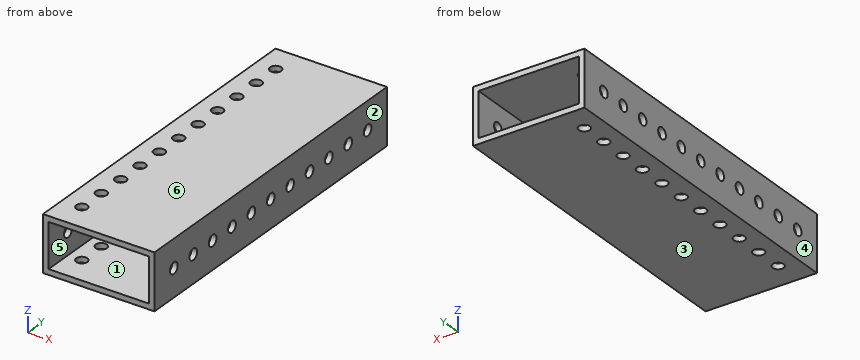
```python
from build123d import *

# Parameters (mm, degrees)
SKETCH1_W           = 50.8
SKETCH1_H           = 25.4
SKETCH1_W_2         = 45.72
SKETCH1_H_2         = 20.32
BOSS_EXTRUDE2_DEPTH = 152.4
SKETCH2_R           = 2.54
CUT_EXTRUDE1_DEPTH  = 127
SKETCH3_R           = 2.54
CUT_EXTRUDE2_DEPTH  = 166.725706651


with BuildPart() as part:
    # Sketch1 → Boss-Extrude2 (new body)
    with BuildSketch(Plane(origin=(0, 0, 0), x_dir=(1, 0, 0), z_dir=(0, 1, 0))):
        with Locations((-34.550728477, 5.021125828)):
            Rectangle(SKETCH1_W, SKETCH1_H)
        with Locations((-34.550728477, 5.021125828)):
            Rectangle(SKETCH1_W_2, SKETCH1_H_2, mode=Mode.SUBTRACT)
    extrude(amount=BOSS_EXTRUDE2_DEPTH)

    # Sketch2 → Cut-Extrude1 (cut)
    with BuildSketch(Plane(origin=(-9.150728477, 0, 0), x_dir=(0, 0, -1), z_dir=(1, 0, 0))):
        with Locations((5.021125828, 139.7)):
            Circle(SKETCH2_R)
        with Locations((5.021125828, 127)):
            Circle(SKETCH2_R)
        with Locations((5.021125828, 114.3)):
            Circle(SKETCH2_R)
        with Locations((5.021125828, 101.6)):
            Circle(SKETCH2_R)
        with Locations((5.021125828, 88.9)):
            Circle(SKETCH2_R)
        with Locations((5.021125828, 76.2)):
            Circle(SKETCH2_R)
        with Locations((5.021125828, 63.5)):
            Circle(SKETCH2_R)
        with Locations((5.021125828, 50.8)):
            Circle(SKETCH2_R)
        with Locations((5.021125828, 38.1)):
            Circle(SKETCH2_R)
        with Locations((5.021125828, 25.4)):
            Circle(SKETCH2_R)
        with Locations((5.021125828, 12.7)):
            Circle(SKETCH2_R)
    extrude(amount=-CUT_EXTRUDE1_DEPTH, mode=Mode.SUBTRACT)

    # Sketch3 → Cut-Extrude2 (cut, through all)
    with BuildSketch(Plane(origin=(0, 0, -17.721125828), x_dir=(-1, 0, 0), z_dir=(0, 0, -1))):
        with Locations((51.060728477, 139.7)):
            Circle(SKETCH3_R)
        with Locations((51.060728477, 127)):
            Circle(SKETCH3_R)
        with Locations((51.060728477, 114.3)):
            Circle(SKETCH3_R)
        with Locations((51.060728477, 101.6)):
            Circle(SKETCH3_R)
        with Locations((51.060728477, 88.9)):
            Circle(SKETCH3_R)
        with Locations((51.060728477, 76.2)):
            Circle(SKETCH3_R)
        with Locations((51.060728477, 63.5)):
            Circle(SKETCH3_R)
        with Locations((51.060728477, 50.8)):
            Circle(SKETCH3_R)
        with Locations((51.060728477, 38.1)):
            Circle(SKETCH3_R)
        with Locations((51.060728477, 25.4)):
            Circle(SKETCH3_R)
        with Locations((51.060728477, 12.7)):
            Circle(SKETCH3_R)
    extrude(amount=-CUT_EXTRUDE2_DEPTH, mode=Mode.SUBTRACT)


solid = part.part
```
The model under review builds one solid part; all positions refer to its coordinate system, in mm. Face numbers are marked on the shaded views. A direction names the side the tool comes from. Round coordinates to 2 decimals unless told otherwise and drop trailing zeros. Loops run counter-clockwise (first coordinate to the right, second up) from the corner with the lowest first, then second, coordinate; pieces in that order, holes last. Notation, with made-up numbers: M 19.5,25.5 L 67.5,25.5 A31 ccw 67.5,60.5 Z; hole C -36,-30.75 d1. An arc over 180 degrees is marked long. Put each result on its own line as item: value.
Q1. To check wall thickness, follow L1, parallel to X at y = 82.5, z = 1; L2, parallel to Z at x = -43, y = 62.5; L3, parallel to Z at x = -58, y = 88. State the ranges of each line that lie inside material, in increasing order.
Result set:
L1: x = -59.95 to -57.41, -11.69 to -9.15
L2: z = -17.72 to -15.18, 5.14 to 7.68
L3: z = -17.72 to -7.4, -2.65 to 7.68
Q2. For pin 1 (8 mm diameter, centred on x = -45, z = 0, fed in from +Y), flat-tipped, find the tip position at first contact; note if it passes through.
Result set:
pin 1: passes through
Q3. Consider section A-A, the plane z = 3.5. Give the boundary of the cut face in (x, y).
Result set:
outline: M -59.95,0 L -57.41,0 L -57.41,152.4 L -59.95,152.4 Z; M -11.69,0 L -9.15,0 L -9.15,152.4 L -11.69,152.4 Z
Q4. Consider section D-D, the plane y = 63.5. Give the boundary of the cut face in (x, z), then the cut area to 3 significant figures.
Result set:
outline: M -59.95,-17.72 L -53.6,-17.72 L -53.6,-15.18 L -57.41,-15.18 L -57.41,-7.56 L -59.95,-7.56 Z; M -59.95,-2.48 L -57.41,-2.48 L -57.41,5.14 L -53.6,5.14 L -53.6,7.68 L -59.95,7.68 Z; M -48.52,-17.72 L -9.15,-17.72 L -9.15,-7.56 L -11.69,-7.56 L -11.69,-15.18 L -48.52,-15.18 Z; M -48.52,5.14 L -11.69,5.14 L -11.69,-2.48 L -9.15,-2.48 L -9.15,7.68 L -48.52,7.68 Z
area: 310 mm²
Q5. Consider section C-C, the plane x = -55. Give the boundary of the cut face in (y, z).
Result set:
outline: M 0,-17.72 L 152.4,-17.72 L 152.4,-15.18 L 0,-15.18 Z; M 0,5.14 L 152.4,5.14 L 152.4,7.68 L 0,7.68 Z
Q6. Machinability: for the marked faces 1 and 2, which of the approach directions +Z, -Z, +X, -X, +Y, -Y give a long, thin tool a straight path to every point of the face, cutting with its end or side? Answer none if there is none.
Result set:
face 1: +Y, -Y
face 2: +Z, -Z, +X, +Y, -Y
Q7. Consider section B-B, the plane y = 19.5. Give the boundary of the cut face in (x, z), then the cut area to 3 significant figures.
Result set:
outline: M -59.95,-17.72 L -9.15,-17.72 L -9.15,7.68 L -59.95,7.68 Z; hole M -57.41,-15.18 L -11.69,-15.18 L -11.69,5.14 L -57.41,5.14 Z
area: 361 mm²
Q8. Mouldability with a two-part tool opening along Z and no side actions: class the marked faces 3, 4, 5 and 6 as released by +Z, released by -Z, zero draft, split by the parting line, or undercut.
Result set:
face 3: released by -Z
face 4: zero draft
face 5: undercut
face 6: released by +Z
